The model under review builds one solid part; all positions refer to its coordinate system, in mm. A direction names the side the tool comes from. Give positions to 0.01 mm unless a question says otherwise; leave off trailing zeros. Write each loop counter-clockwise with the first axis right and the second up, starting at its lowest first coordinate (ties: lowest second). Pieces come first, ordered by that corner, then holes. Notation, with made-up numbers: (46, -11.5) - (90, -11.5) arc R17 cw to (90, 20.5) - close; hole circle Ø9 at (68.5, 71). An arc over 180 degrees is marked (long way). One line per question, with ' | ' between items. Start each with the question number.
```python
from build123d import *

# Parameters (mm, degrees)
SKETCH1_W                = 40
SKETCH1_H                = 10
BOSS_EXTRUDE1_DEPTH      = 3
BOSS_EXTRUDE2_DEPTH      = 5
BOSS_EXTRUDE2_DEPTH_BACK = 5
FILLET1_START            = -6
FILLET1_DEPTH            = 12
M4_CLEARANCE_HOLE1_D     = 4.5


with BuildPart() as part:
    # Sketch1 → Boss-Extrude1 (new body)
    with BuildSketch(Plane(origin=(0, 0, 0), x_dir=(1, 0, 0), z_dir=(0, 1, 0))):
        Rectangle(SKETCH1_W, SKETCH1_H)
    extrude(amount=BOSS_EXTRUDE1_DEPTH)

    # Sketch2 → Boss-Extrude2 (add, two sides: drawn at the far end of the back side and taken through both)
    with BuildSketch(Plane.XY.offset(-BOSS_EXTRUDE2_DEPTH_BACK)):
        with BuildLine():
            Line((11.25, 15.5), (11.25, 3))
            Line((11.25, 3), (-11.25, 3))
            Line((-11.25, 3), (-11.25, 15.5))
            ThreePointArc((-11.25, 15.5), (0, 4.25), (11.25, 15.5))
        make_face()
    extrude(amount=BOSS_EXTRUDE2_DEPTH + BOSS_EXTRUDE2_DEPTH_BACK)

    # Fillet1: read off the stored shape, not the designer's step
    # Fillet1 outline → Fillet1 (cut)
    with BuildSketch(Plane.XY.offset(FILLET1_START)):
        with BuildLine():
            ThreePointArc((11.25, 15.5), (10.781042034, 12.285714286), (9.413265306, 9.339404552))
            ThreePointArc((9.413265306, 9.339404552), (10.535714285, 9.750110915), (11.25, 8.791796068))
            Line((11.25, 8.791796068), (11.25, 15.5))
        make_face()
        with BuildLine():
            ThreePointArc((-11.25, 8.791796068), (-10.535714285, 9.750110915), (-9.413265306, 9.339404552))
            ThreePointArc((-9.413265306, 9.339404552), (-10.781042034, 12.285714286), (-11.25, 15.5))
            Line((-11.25, 15.5), (-11.25, 8.791796068))
        make_face()
    extrude(amount=FILLET1_DEPTH, mode=Mode.SUBTRACT)

    # M4 Clearance Hole1 (through all)
    with Locations(Plane(origin=(0, 0, 0), x_dir=(-1, 0, 0), z_dir=(0, -1, 0))):
        with Locations((15, 0), (-15, 0)):
            Hole(M4_CLEARANCE_HOLE1_D / 2)


solid = part.part
```
Item 1: Clearance check with flat-ended pins moving along their axes: P1, Ø3, axis at y = 6.5, z = -1, coming from the -X side; P2, Ø5, axis at x = 15, z = 0, coming from the +Y side; P3, Ø4.5, axis at y = 7, z = -0.5, coming from the +X side. State where each tip first meets the part, or that it passes through.
Item 2: Take a section at B-B (y = 1). Give the boundary of the cut face in (x, z), plus the area to 3 significant figures.
Item 3: For probe 1 along Z at (x, y) = (-15, 2.2); probe 2 along X at (y, z) = (1.25, 1); probe 3 along X at (y, z) = (3.5, -1.75), list the stretches that pass through material, from the lowest coordinate up.
Item 4: Take a section at D-D (y = 5). Give the boundary of the cut face in (x, z), plus the area to 3 significant figures.
Item 5: Take a section at A-A (x = -15). Give the boundary of the cut face in (y, z).
Item 6: The part is to be moulded in two halves that separate along X. For faces 4 (the flat face through (0, 3, 5)), 5 (the cylindrical face through (-0.16, 4.25, -0.07)), 6 (the flat face through (-20, 1, 0)), 7 (the cylindrical face through (17.146, 1.521, -0.676)), say which applies: +X half, -X half, draft (parallel to the pull), parting line (faces both ways), or undercut.
Item 7: Take a section at C-C (z = 0). Give the boundary of the cut face in (x, y).
Item 8: Machinability: for faces 1 (the flat face through (-18, 3, 0)), 2 (the flat face through (0, 3, -5)), 3 (the flat face through (11.25, 6, 0)), which of the approach directions +Z, -Z, +X, -X, +Y, -Y give a long, thin tool a straight path to every point of the face, cutting with its end or side? Answer none if there is none.
Check sheet entries:
1) P1: stops at x = -11.25 | P2: stops at y = 3 | P3: stops at x = 11.25
2) outline: (-20, -5) - (20, -5) - (20, 5) - (-20, 5) - close; hole circle Ø4.5 at (-15, 0); hole circle Ø4.5 at (15, 0) | area: 368 mm^2
3) probe 1: z = -5 to -2.25, 2.25 to 5 | probe 2: x = -20 to -17.02, -12.98 to 12.98, 17.02 to 20 | probe 3: x = -11.25 to 11.25
4) outline: (-11.25, -5) - (-4.04, -5) - (-4.04, 5) - (-11.25, 5) - close; (4.04, -5) - (11.25, -5) - (11.25, 5) - (4.04, 5) - close | area: 144 mm^2
5) outline: (0, -5) - (3, -5) - (3, -2.25) - (0, -2.25) - close; (0, 2.25) - (3, 2.25) - (3, 5) - (0, 5) - close
6) face 4: draft | face 5: undercut | face 6: -X half | face 7: undercut
7) outline: (-20, 0) - (-17.25, 0) - (-17.25, 3) - (-20, 3) - close; (-12.75, 0) - (12.75, 0) - (12.75, 3) - (11.25, 3) - (11.25, 8.79) arc R1 ccw to (9.41, 9.34) arc R11.25 cw to (-9.41, 9.34) arc R1 ccw to (-11.25, 8.79) - (-11.25, 3) - (-12.75, 3) - close; (17.25, 0) - (20, 0) - (20, 3) - (17.25, 3) - close
8) face 1: +Z, -Z, -X, +Y | face 2: -Z, +X, -X, +Y, -Y | face 3: +Z, -Z, +X, +Y
